Model file for the job. Use its own axes, mm. A direction names the side the tool comes from. Give positions to 0.01 mm unless a question says otherwise; leave off trailing zeros. Order: outer loops, then holes, each group sorted by start corner. A loop starts at its lowest first (then second) coordinate and runs counter-clockwise, first axis right, second up. Notation, with made-up numbers: M 48,40 L 71,40 A22 ccw 71,72 Z; hole C 81,45 d8. An arc over 180 degrees is marked long. Return JSON: item names as keys, results as strings. Group by question number.
1. Slice it at B-B on y = -6.75. List the corners of the cut face in (x, z), then the cut area to 3 significant figures.
2. Wall check: probe 1 along Y at (x, z) = (22, 1); probe 2 along X at (y, z) = (-0.75, 0); probe 3 along X at (y, z) = (-5.25, 18.5). Give the ranges that are in metal, low to high. Write a range as [from, to].
3. Slice it at C-C on x = -27.5. List the corners of the cut face in (y, z).
4. 3-axis set-ups, long thin cutter, end or side, ignore diameter. For faces 1 (the face through (-33.54, -4.93, 0.47)), 2 (the face through (36, 0, -1)): which of +Z, -Z, +X, -X, +Y, -Y reach the whole face in a straight line?
5. Slice it at D-D on z = -36. List the corners of the cut face in (x, y), then the cut area to 3 significant figures.
6. Two-plate mould, pull along Z, no slides. Class faces 3 (the face through (0, 0, 0)), 4 (the face through (-31.114, -6, 0.439)), 5 (the face through (-1, 3, -1)), 6 (the face through (-0.47, -4.93, -33.54)): released by +Z, released by -Z, zero draft, split by the parting line, or undercut.
7. Slice it at A-A on z = -16. List the corners of the cut face in (x, y).
8. Pin check, flat tips, straight feed: pin 1 (12 mm diameter, centred on x = 7.5, z = -3.5, fed in from -Y); pin 2 (2 mm diameter, centred on x = 11, y = -4, fed in from +Z); pin 3 (4 mm diameter, centred on x = -31, y = -5, fed in from -Z). Stop position of each tip, or through.
from build123d import *

# Parameters (mm, degrees)
SKETCH1_W             = 67.6
SKETCH1_H             = 67.6
SKETCH1_W_2           = 61.6
SKETCH1_H_2           = 61.6
BOSS_EXTRUDE1_DEPTH   = 10
BOSS_EXTRUDE1_DRAFT   = -3
SKETCH2_W             = 83
SKETCH2_H             = 83
BOSS_EXTRUDE2_DEPTH   = 3
CHAMFER1_SIZE         = 1.5
CHAMFER2_SIZE         = 2
CHAMFER2_SIZE2        = 2.113509005
CHAMFER2_EDGE_2_SIZE  = 2
CHAMFER2_EDGE_2_SIZE2 = 2.113509005
CHAMFER2_EDGE_3_SIZE  = 2
CHAMFER2_EDGE_3_SIZE2 = 2.113509005
CHAMFER2_EDGE_4_SIZE  = 2
CHAMFER2_EDGE_4_SIZE2 = 2.113509005


with BuildPart() as part:
    # Sketch1 → Boss-Extrude1 (with draft: the straight prism first)
    with BuildSketch(Plane(origin=(0, 0, 0), x_dir=(1, 0, 0), z_dir=(0, 1, 0))):
        Rectangle(SKETCH1_W, SKETCH1_H)
        Rectangle(SKETCH1_W_2, SKETCH1_H_2, mode=Mode.SUBTRACT)
    extrude(amount=-BOSS_EXTRUDE1_DEPTH)
    # Boss-Extrude1: the draft: its side faces are tilted about the plane it starts from
    boss_extrude1_sides = [part.faces().sort_by_distance(p)[0] for p in [
        (-33.8, -5, 0),
        (0, -5, 33.8),
        (33.8, -5, 0),
        (0, -5, -33.8),
        (0, -5, -30.8),
        (30.8, -5, 0),
        (0, -5, 30.8),
        (-30.8, -5, 0),
    ]]
    draft(boss_extrude1_sides, Plane(origin=(0, 0, 0), x_dir=(1, 0, 0), z_dir=(0, 1, 0)), BOSS_EXTRUDE1_DRAFT)

    # Sketch2 → Boss-Extrude2 (add)
    with BuildSketch(Plane(origin=(0, 0, 0), x_dir=(1, 0, 0), z_dir=(0, 1, 0))):
        Rectangle(SKETCH2_W, SKETCH2_H)
    extrude(amount=BOSS_EXTRUDE2_DEPTH)

    # Chamfer1
    chamfer1_edges = [part.edges().sort_by_distance(p)[0] for p in [
        (41.5, 3, 0),
        (0, 3, -41.5),
        (-41.5, 3, 0),
        (0, 3, 41.5),
    ]]
    chamfer(chamfer1_edges, length=CHAMFER1_SIZE)

    # Chamfer2
    chamfer2_edges = [part.edges().sort_by_distance(p)[0] for p in [
        (-30.8, 0, 0),
    ]]
    chamfer2_side = [part.faces().sort_by_distance(p)[0] for p in [
        (0, 0, 0),
    ]]
    chamfer(chamfer2_edges, length=CHAMFER2_SIZE, length2=CHAMFER2_SIZE2, reference=chamfer2_side[0])

    # Chamfer2 edge 2
    chamfer2_edge_2_edges = [part.edges().sort_by_distance(p)[0] for p in [
        (0, 0, 30.8),
    ]]
    chamfer2_edge_2_side = [part.faces().sort_by_distance(p)[0] for p in [
        (0, 0, 0),
    ]]
    chamfer(chamfer2_edge_2_edges, length=CHAMFER2_EDGE_2_SIZE, length2=CHAMFER2_EDGE_2_SIZE2, reference=chamfer2_edge_2_side[0])

    # Chamfer2 edge 3
    chamfer2_edge_3_edges = [part.edges().sort_by_distance(p)[0] for p in [
        (30.8, 0, 0),
    ]]
    chamfer2_edge_3_side = [part.faces().sort_by_distance(p)[0] for p in [
        (0, 0, 0),
    ]]
    chamfer(chamfer2_edge_3_edges, length=CHAMFER2_EDGE_3_SIZE, length2=CHAMFER2_EDGE_3_SIZE2, reference=chamfer2_edge_3_side[0])

    # Chamfer2 edge 4
    chamfer2_edge_4_edges = [part.edges().sort_by_distance(p)[0] for p in [
        (0, 0, -30.8),
    ]]
    chamfer2_edge_4_side = [part.faces().sort_by_distance(p)[0] for p in [
        (0, 0, 0),
    ]]
    chamfer(chamfer2_edge_4_edges, length=CHAMFER2_EDGE_4_SIZE, length2=CHAMFER2_EDGE_4_SIZE2, reference=chamfer2_edge_4_side[0])


solid = part.part
Result:
{
 "1": {"outline": "M -33.45,-33.45 L 33.45,-33.45 L 33.45,33.45 L -33.45,33.45 Z; hole M -31.15,-31.15 L 31.15,-31.15 L 31.15,31.15 L -31.15,31.15 Z", "area": "592 mm2"},
 "2": {"probe 1": "y = [0, 3]", "probe 2": "x = [-33.76, -29.55], [29.55, 33.76]", "probe 3": "x = [-33.52, -31.08], [31.08, 33.52]"},
 "3": {"outline": "M -10,-33.28 L 0,-33.8 L 0,-41.5 L 1.5,-41.5 L 3,-40 L 3,40 L 1.5,41.5 L 0,41.5 L 0,33.8 L -10,33.28 L -10,31.32 L -2.11,30.91 L 0,28.8 L 0,-28.8 L -2.11,-30.91 L -10,-31.32 Z"},
 "4": {"face 1": "+Z, -Z, -X, -Y", "face 2": "-Y"},
 "5": {"outline": "M -41.5,0 L 41.5,0 L 41.5,1.5 L 40,3 L -40,3 L -41.5,1.5 Z", "area": "247 mm2"},
 "6": {"face 3": "undercut", "face 4": "undercut", "face 5": "zero draft", "face 6": "released by -Z"},
 "7": {"outline": "M -41.5,0 L -33.8,0 L -33.28,-10 L -31.32,-10 L -30.91,-2.11 L -28.8,0 L 28.8,0 L 30.91,-2.11 L 31.32,-10 L 33.28,-10 L 33.8,0 L 41.5,0 L 41.5,1.5 L 40,3 L -40,3 L -41.5,1.5 Z"},
 "8": {"pin 1": "stops at y = 0", "pin 2": "stops at z = 33.64", "pin 3": "stops at z = -33.64"}
}
